Part model, mm, in its own coordinate system. A direction names the side the tool comes from. Round coordinates to 2 decimals unless told otherwise and drop trailing zeros. Loops run counter-clockwise (first coordinate to the right, second up) from the corner with the lowest first, then second, coordinate; pieces in that order, holes last.
(1) Cut at C-C on z = 0.85. Count the separate pieces of the cut face and the enclosed holes in it, then the cut area to 3 significant figures.
(2) Mould opens along Y. For faces 3 (the face through (21.5, 0, 0)), 4 (the face through (0, -21, 0)), 5 (the face through (-15, 12.7, -1)) say: +Y half, -Y half, draft (parallel to the pull), parting line (faces both ways), or undercut.
(3) Cut at B-B on y = -16. List the corners of the cut face in (x, z), then the cut area to 3 significant figures.
(4) Flat gauge pin, fed straight in: pin 1 (4.5 mm diameter, centred on x = -15.5, y = 15.5, fed in from -Z). Where does the tip first touch, or does it go through?
(5) Probe probe 1 along Y at (x, z) = (-15.5, -0.4); probe 2 along Y at (x, z) = (16, -0.05); probe 3 along Y at (x, z) = (-15.5, 0.75). List the from-to ranges inside material, lowest first.
(6) Tool access for faces 1 (the face through (17.914, -14.08, -0.76)), 2 (the face through (-14.7, 14, 0.7)): list every direction of +Z, -Z, +X, -X, +Y, -Y with a clear straight run to the whole face (end or side of a thin tool).
(7) Cut at A-A on x = -15.5. List the corners of the cut face in (y, z), then the cut area to 3 significant figures.
from build123d import *

# Parameters (mm, degrees)
SKETCH_W         = 43
SKETCH_H         = 42
SKETCH_R         = 6.2
SKETCH_R_2       = 1.7
PAD_DEPTH        = 1.5
HOLE_D           = 3.3
HOLE_CSINK_D     = 6
HOLE_CSINK_ANGLE = 90
POCKET_DEPTH     = 1.5
CHAMFER_SIZE     = 4


with BuildPart() as part:
    # Sketch → Pad (new body, symmetric)
    with BuildSketch(Plane.XY):
        Rectangle(SKETCH_W, SKETCH_H)
        Circle(SKETCH_R, mode=Mode.SUBTRACT)
        with Locations((-15.5, 15.5)):
            Circle(SKETCH_R_2, mode=Mode.SUBTRACT)
        with Locations((15.5, 15.5)):
            Circle(SKETCH_R_2, mode=Mode.SUBTRACT)
        with Locations((-15.5, -15.5)):
            Circle(SKETCH_R_2, mode=Mode.SUBTRACT)
        with Locations((15.5, -15.5)):
            Circle(SKETCH_R_2, mode=Mode.SUBTRACT)
    extrude(amount=PAD_DEPTH, both=True)

    # Hole (through all)
    with Locations(Plane.XY.offset(1.5)):
        with Locations((15.909903, -6.010408), (0.938052, -10.022103), (-6.010408, 15.909903), (-10.022103, 0.938052)):
            CounterSinkHole(HOLE_D / 2, HOLE_CSINK_D / 2, counter_sink_angle=HOLE_CSINK_ANGLE)

    # Sketch004 (on Face4 of Hole) → Pocket (cut)
    with BuildSketch(Plane(origin=(0, 0, -1.5), x_dir=(1, 0, 0), z_dir=(0, 0, -1))):
        Polygon((-13.883419, 12.7), (-12.266838, 15.5), (-13.883419, 18.3), (-17.116581, 18.3), (-18.733162, 15.5), (-17.116581, 12.7), align=None)
        Polygon((13.883419, 12.7), (17.116581, 12.7), (18.733162, 15.5), (17.116581, 18.3), (13.883419, 18.3), (12.266838, 15.5), align=None)
        Polygon((17.116581, -12.7), (13.883419, -12.7), (12.266838, -15.5), (13.883419, -18.3), (17.116581, -18.3), (18.733162, -15.5), align=None)
        Polygon((-13.883419, -12.7), (-17.116581, -12.7), (-18.733162, -15.5), (-17.116581, -18.3), (-13.883419, -18.3), (-12.266838, -15.5), align=None)
    extrude(amount=-POCKET_DEPTH, mode=Mode.SUBTRACT)

    # Chamfer
    chamfer_edges = [part.edges().sort_by_distance(p)[0] for p in [
        (21.5, -21, 0),
        (21.5, 21, 0),
        (-21.5, 21, 0),
        (-21.5, -21, 0),
    ]]
    chamfer(chamfer_edges, length=CHAMFER_SIZE)


solid = part.part
Final values:
1. separate pieces: 1
1. enclosed holes: 9
1. area: 1,550 mm2
2. face 3: draft
2. face 4: -Y half
2. face 5: undercut
3. outline: (-21.5, -1.5) - (-18.44, -1.5) - (-18.44, 0) - (-17.12, 0) - (-17.12, 1.5) - (-21.5, 1.5) - close; (-13.88, 0) - (-12.56, 0) - (-12.56, -1.5) - (12.56, -1.5) - (12.56, 0) - (13.88, 0) - (13.88, 1.5) - (-13.88, 1.5) - close; (17.12, 0) - (18.44, 0) - (18.44, -1.5) - (21.5, -1.5) - (21.5, 1.5) - (17.12, 1.5) - close
3. area: 102 mm2
4. pin 1: stops at z = 0
5. probe 1: y = -21 to -18.3, -12.7 to 12.7, 18.3 to 21
5. probe 2: y = -21 to -18.3, -12.7 to -7.66, -4.36 to 12.7, 18.3 to 21
5. probe 3: y = -21 to -17.2, -13.8 to 13.8, 17.2 to 21
6. face 1: -Z
6. face 2: +Z, -Z
7. outline: (-21, -1.5) - (-18.3, -1.5) - (-18.3, 0) - (-17.2, 0) - (-17.2, 1.5) - (-21, 1.5) - close; (-13.8, 0) - (-12.7, 0) - (-12.7, -1.5) - (12.7, -1.5) - (12.7, 0) - (13.8, 0) - (13.8, 1.5) - (-13.8, 1.5) - close; (17.2, 0) - (18.3, 0) - (18.3, -1.5) - (21, -1.5) - (21, 1.5) - (17.2, 1.5) - close
7. area: 99.0 mm2
